Model file for the job. Use its own axes, mm. A direction names the side the tool comes from. Round coordinates to 2 decimals unless told otherwise and drop trailing zeros. Order: outer loops, then holes, each group sorted by start corner. A loop starts at its lowest first (then second) coordinate and runs counter-clockwise, first axis right, second up. Notation, with made-up numbers: (59, 61) -> (118, 61) arc R33 cw to (118, 89) -> close; hole circle Ø4 at (-36, 73). An arc over 180 degrees is marked (long way). Put each result on its own line as item: value. Start each with the question number.
Q1. Flat gauge pins, fed straight in: P1, Ø5, axis at x = -0.5, z = 4.5, coming from the -Y side; P2, Ø2.5, axis at x = 0.5, z = 0.5, coming from the -Y side; P3, Ø3, axis at x = 0.37, z = 1.33, coming from the +Y side. Where does each tip first touch, or does it go through?
Q2. 3-axis set-ups, long thin cutter, end or side, ignore diameter. For faces 1 (the face through (-7, 0, 1)), 2 (the face through (-6.035, 4, 1)), 3 (the face through (-4.58, 10.34, 7.64)): which of +Z, -Z, +X, -X, +Y, -Y reach the whole face in a straight line?
Q3. Cut at A-A, the plane y = 3.5. List the corners of the cut face in (x, z) (3 decimals), and give its area (3 significant figures).
Q4. Cut at B-B, the plane y = 10. List the corners of the cut face in (x, z).
Q5. Pull direction Z, two halves, no side cores. Call faces 4 (the face through (8.275, 4, 1)), 5 (the face through (0, 4, -6.572)), 6 (the face through (-3, 8.1, 3)): released by +Z, released by -Z, zero draft, split by the parting line, or undercut.
Q6. Probe L1, parallel to Z at x = -4.5, y = 1.5; L2, parallel to Z at x = 1.75, y = 3.5; L3, parallel to X at y = 1.25, z = 1.75. List the from-to ranges inside material, lowest first.
from build123d import *

# Parameters (mm, degrees)
SKETCH1_W              = 15.8
SKETCH1_H              = 15.8
BOSS_EXTRUDE1_DEPTH    = 9.6
FILLET1_R              = 0.5
SKETCH2_W              = 12.82
SKETCH2_H              = 12.82
CUT_EXTRUDE1_DEPTH     = 8.1
SKETCH3_R              = 2.5
BOSS_EXTRUDE2_DEPTH    = 1.7
FILLET2_R              = 0.2
LPATTERN1_COUNT        = 2
LPATTERN1_PITCH        = 8
LPATTERN1_COUNT_DIR2   = 2
LPATTERN1_PITCH_DIR2   = 8
FILLET2_OF_LPATTERN1_R = 0.2
SKETCH4_R              = 3.155
BOSS_EXTRUDE3_DEPTH    = 8.1
SKETCH5_R              = 2.655
CUT_EXTRUDE2_DEPTH     = 8.1


with BuildPart() as part:
    # Sketch1 → Boss-Extrude1 (new body)
    with BuildSketch(Plane(origin=(0, 0, 0), x_dir=(1, 0, 0), z_dir=(0, 1, 0))):
        with Locations((0.374568966, -1.328017241)):
            Rectangle(SKETCH1_W, SKETCH1_H)
    extrude(amount=BOSS_EXTRUDE1_DEPTH)

    # Fillet1
    fillet1_edges = [part.edges().sort_by_distance(p)[0] for p in [
        (8.274568966, 9.6, 1.328017241),
        (0.374568966, 9.6, -6.571982759),
        (-7.525431034, 9.6, 1.328017241),
        (0.374568966, 9.6, 9.228017241),
        (-7.525431034, 4.8, -6.571982759),
        (8.274568966, 4.8, -6.571982759),
        (8.274568966, 4.8, 9.228017241),
        (-7.525431034, 4.8, 9.228017241),
    ]]
    fillet(fillet1_edges, radius=FILLET1_R)

    # Sketch2 → Cut-Extrude1 (cut)
    with BuildSketch(Plane.XZ):
        with Locations((0.374568966, 1.328017241)):
            Rectangle(SKETCH2_W, SKETCH2_H)
    extrude(amount=-CUT_EXTRUDE1_DEPTH, mode=Mode.SUBTRACT)

    # Sketch3 → Boss-Extrude2 (add)
    with BuildSketch(Plane(origin=(0, 9.6, 0), x_dir=(1, 0, 0), z_dir=(0, 1, 0))):
        with Locations(Location((-3.625431034, 2.671982759, 0), (0, 0, 270))):
            Circle(SKETCH3_R)
    boss_extrude2 = extrude(amount=BOSS_EXTRUDE2_DEPTH)

    # Fillet2
    fillet2_edges = [part.edges().sort_by_distance(p)[0] for p in [
        (-3.625431034, 11.3, -5.171982759),
    ]]
    fillet(fillet2_edges, radius=FILLET2_R)

    # LPattern1: Boss-Extrude2 2 × 2
    with Locations(*[(i * LPATTERN1_PITCH, 0, j * LPATTERN1_PITCH_DIR2) for i in range(LPATTERN1_COUNT) for j in range(LPATTERN1_COUNT_DIR2) if (i, j) != (0, 0)]):
        add(boss_extrude2)

    # Fillet2 of LPattern1
    fillet2_of_lpattern1_edges = [part.edges().sort_by_distance(p)[0] for p in [
        (-3.625431034, 11.3, 2.828017241),
        (4.374568966, 11.3, -5.171982759),
        (4.374568966, 11.3, 2.828017241),
    ]]
    fillet(fillet2_of_lpattern1_edges, radius=FILLET2_OF_LPATTERN1_R)

    # Sketch4 → Boss-Extrude3 (add)
    with BuildSketch(Plane.XZ.offset(-8.1)):
        with Locations(Location((0.374568966, 1.328017241, 0), (0, 0, 90))):
            Circle(SKETCH4_R)
    extrude(amount=BOSS_EXTRUDE3_DEPTH)

    # Sketch5 → Cut-Extrude2 (cut)
    with BuildSketch(Plane.XZ):
        with Locations(Location((0.374568966, 1.328017241, 0), (0, 0, 270))):
            Circle(SKETCH5_R)
    extrude(amount=-CUT_EXTRUDE2_DEPTH, mode=Mode.SUBTRACT)


solid = part.part
Ans:
1. P1: stops at y = 0
1. P2: stops at y = 8.1
1. P3: stops at y = 9.6
2. face 1: +Z, -Z, +X, -X, -Y
2. face 2: -Y
2. face 3: +Y
3. outline: (-7.525, -6.072) arc R0.5 ccw to (-7.025, -6.572) -> (7.775, -6.572) arc R0.5 ccw to (8.275, -6.072) -> (8.275, 8.728) arc R0.5 ccw to (7.775, 9.228) -> (-7.025, 9.228) arc R0.5 ccw to (-7.525, 8.728) -> close; circle Ø6.31 at (0.375, 1.328); hole (-6.035, -5.082) -> (6.785, -5.082) -> (6.785, 7.738) -> (-6.035, 7.738) -> close; hole circle Ø5.31 at (0.375, 1.328)
3. area: 94.2 mm^2
4. outline: circle Ø5 at (-3.63, -2.67); circle Ø5 at (-3.63, 5.33); circle Ø5 at (4.37, -2.67); circle Ø5 at (4.37, 5.33)
5. face 4: zero draft
5. face 5: released by -Z
5. face 6: undercut
6. L1: z = -6.57 to -5.08, 7.74 to 9.23
6. L2: z = -6.57 to -5.08, -1.51 to -0.94, 3.6 to 4.17, 7.74 to 9.23
6. L3: x = -7.53 to -6.04, -2.75 to -2.25, 3 to 3.5, 6.78 to 8.27
